Geometry check sheet. Reference: drawing and pictorial views, mm from the part's lowest x, y, z. A direction names the side the tool comes from. Give positions to 0.01 mm unless a question says otherwise; leave off trailing zeros. Order: outer loops, then holes, each group sorted by start corner. A loop starts at its lowest first (then second) coordinate and runs counter-clockwise, first axis right, second up. Notation, with made-up numbers: (58, 17.5) - (107, 17.5) arc R15 cw to (107, 21.5) - close; hole circle Ø8 at (45.5, -27). An arc over 180 degrees is marked (long way). Answer as a JSON object with one key per item and string values.
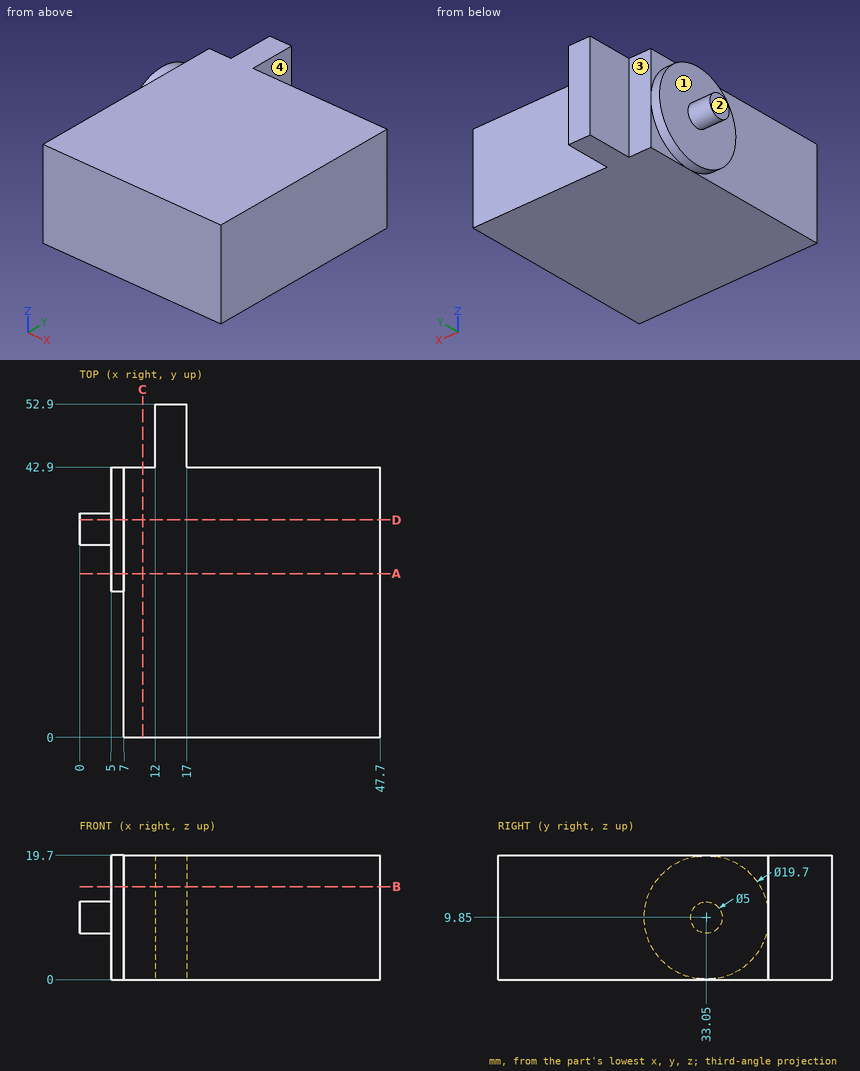
(1) Access from +Z, -Z, +X, -X, +Y, -Y to the whole of each face (thin tool, end or side, straight path). Record for the marked faces 1, 2, 3 and 4.
Computed values:
{"face 1": "-X", "face 2": "+Z, -Z, -X, +Y, -Y", "face 3": "+Z, -Z, -X, +Y", "face 4": "+Z, -Z, +X, +Y"}
(2) Section check C-C (x = 10). Record the cut outline in (y, z).
Computed values:
{"outline": "(0, 0) - (42.9, 0) - (42.9, 19.7) - (0, 19.7) - close"}
(3) Section check B-B (z = 14.75). Record the cut outline in (x, y), then the cut area to 3 significant figures.
Computed values:
{"outline": "(5, 24.51) - (7, 24.51) - (7, 0) - (47.7, 0) - (47.7, 42.9) - (17, 42.9) - (17, 52.9) - (12, 52.9) - (12, 42.9) - (7, 42.9) - (7, 41.59) - (5, 41.59) - close", "area": "1,830 mm²"}
(4) Section check A-A (y = 26). Record the cut outline in (x, z), then the cut area to 3 significant figures.
Computed values:
{"outline": "(5, 2.97) - (7, 2.97) - (7, 0) - (47.7, 0) - (47.7, 19.7) - (7, 19.7) - (7, 16.73) - (5, 16.73) - close", "area": "829 mm²"}
(5) Material ranges on line 1 along Y through (x, z) = (17.5, 7.5); line 2 along X through (y, z) = (24.5, 7.75); line 3 along X through (y, z) = (4, 12.5), recorded low to high. Write a range as [from, to].
Computed values:
{"line 1": "y = [0, 42.9]", "line 2": "x = [5, 47.7]", "line 3": "x = [7, 47.7]"}
(6) Gauge pin test, flat ends, axial feed: pin 1 Ø3 at (x, z) = (42, 11.5) entering from +Y; pin 2 Ø8 at (y, z) = (46.5, 5.5) entering from -X; pin 3 Ø8 at (y, z) = (48.5, 13.5) entering from +X. Record the tip position at first contact, or that the pin passes through.
Computed values:
{"pin 1": "stops at y = 42.9", "pin 2": "stops at x = 7", "pin 3": "stops at x = 17"}
(7) Section check D-D (y = 34.5). Record the cut outline in (x, z).
Computed values:
{"outline": "(0, 7.81) - (5, 7.81) - (5, 0.11) - (7, 0.11) - (7, 0) - (47.7, 0) - (47.7, 19.7) - (7, 19.7) - (7, 19.59) - (5, 19.59) - (5, 11.89) - (0, 11.89) - close"}
